from build123d import *

# Parameters (mm, degrees)
SKETCH1_R           = 38.1635
SKETCH1_R_2         = 13.716
BOSS_EXTRUDE3_DEPTH = 64.262
SKETCH3_R           = 38.1
SKETCH3_R_2         = 14.097
CUT_EXTRUDE1_DEPTH  = 62.23
FILLET1_R           = 2.54
SKETCH5_R           = 2.093695025
SKETCH5_R_2         = 2.032
SKETCH5_R_3         = 2.54
CUT_EXTRUDE2_DEPTH  = 2.54


with BuildPart() as part:
    # Sketch1 → Boss-Extrude3 (new body)
    with BuildSketch(Plane(origin=(0, 0, 0), x_dir=(1, 0, 0), z_dir=(0, 1, 0))):
        with Locations(Location((0, 0, 0), (0, 0, 270))):
            Circle(SKETCH1_R)
        with Locations(Location((0, 0, 0), (0, 0, 270))):
            Circle(SKETCH1_R_2, mode=Mode.SUBTRACT)
    extrude(amount=BOSS_EXTRUDE3_DEPTH)

    # Sketch3 → Cut-Extrude1 (cut)
    with BuildSketch(Plane(origin=(0, 0, 0), x_dir=(-1, 0, 0), z_dir=(0, -1, 0))):
        with Locations(Location((0, 0, 0), (0, 0, 90))):
            Circle(SKETCH3_R)
        with Locations(Location((0, 0, 0), (0, 0, 90))):
            Circle(SKETCH3_R_2, mode=Mode.SUBTRACT)
    extrude(amount=-CUT_EXTRUDE1_DEPTH, mode=Mode.SUBTRACT)

    # Fillet1
    fillet1_edges = [part.edges().sort_by_distance(p)[0] for p in [
        (0, 64.262, -38.1635),
        (0, 64.262, -13.716),
    ]]
    fillet(fillet1_edges, radius=FILLET1_R)

    # Sketch5 → Cut-Extrude2 (cut)
    with BuildSketch(Plane(origin=(0, 64.262, 0), x_dir=(1, 0, 0), z_dir=(0, 1, 0))):
        with Locations(Location((15.256423447, 20.307672038, 0), (0, 0, 270))):
            Circle(SKETCH5_R)
        with Locations(Location((-25.2151716, 3.058614257, 0), (0, 0, 270))):
            Circle(SKETCH5_R_2)
        with Locations(Location((9.958748153, -23.366286295, 0), (0, 0, 270))):
            Circle(SKETCH5_R_2)
        with Locations(Location((-9.958748153, 23.366286295, 0), (0, 0, 270))):
            Circle(SKETCH5_R_3)
    extrude(amount=-CUT_EXTRUDE2_DEPTH, mode=Mode.SUBTRACT)


solid = part.part
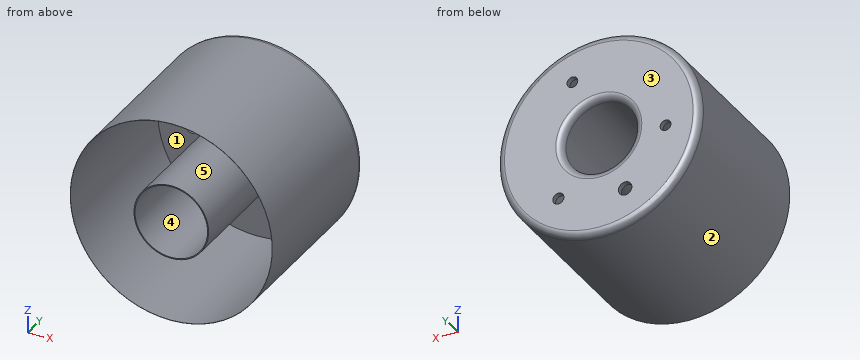
Check sheet for the modelled part. Datum: model origin and axes. Units: mm. Face numbers are marked on the shaded views. A direction names the side the tool comes from. Round coordinates to 2 decimals unless told otherwise and drop trailing zeros. Order: outer loops, then holes, each group sorted by start corner. A loop starts at its lowest first (then second) coordinate and runs counter-clockwise, first axis right, second up.
(1) Cross-section at B-B, the plane x = 0. Enter the section's corners in (y, z).
(2) Cross-section at A-A, the plane z = 0. Enter the section's corners in (x, y), and give its area (3 significant figures).
(3) Scan lines: probe 1 along Y at (x, z) = (26, 19); probe 2 along Z at (x, y) = (-35, 11). Record each from-to range of solid material in increasing order.
(4) Draft check along Z on the marked faces 1, 2 and 3. Enter one of: pulls with the +Z half, pulls with the -Z half, needs draft (parallel to the pull), parting line crosses it, or undercut.
(5) Go/stop test with flat-tipped pins: P1, Ø12, axis at x = -24.5, y = 34, coming from the -Z side; P2, Ø2, axis at x = 29.5, y = 6.5, coming from the -Z side; P3, Ø5, axis at x = -4, y = 45.5, coming from the +Z side. Record where each tip stops, or that it passes through.
(6) Cross-section at C-C, the plane y = 11.5. Enter the section's corners in (x, z).
(7) Access from +Z, -Z, +X, -X, +Y, -Y to the whole of each face (thin tool, end or side, straight path). Record for the marked faces 4 and 5.
Check sheet entries:
1. outline: (0, -38.16) - (61.72, -38.16) arc R2.54 ccw to (64.26, -35.62) - (64.26, -16.26) arc R2.54 ccw to (61.72, -13.72) - (0, -13.72) - (0, -14.1) - (62.23, -14.1) - (62.23, -38.1) - (0, -38.1) - close; (0, 13.72) - (61.72, 13.72) arc R2.54 ccw to (64.26, 16.26) - (64.26, 35.62) arc R2.54 ccw to (61.72, 38.16) - (0, 38.16) - (0, 38.1) - (62.23, 38.1) - (62.23, 14.1) - (0, 14.1) - close
2. outline: (-38.16, 0) - (-38.1, 0) - (-38.1, 62.23) - (-14.1, 62.23) - (-14.1, 0) - (-13.72, 0) - (-13.72, 61.72) arc R2.54 ccw to (-16.26, 64.26) - (-35.62, 64.26) arc R2.54 ccw to (-38.16, 61.72) - close; (13.72, 0) - (14.1, 0) - (14.1, 62.23) - (38.1, 62.23) - (38.1, 0) - (38.16, 0) - (38.16, 61.72) arc R2.54 ccw to (35.62, 64.26) - (16.26, 64.26) arc R2.54 ccw to (13.72, 61.72) - close
2. area: 149 mm2
3. probe 1: y = 62.23 to 64.26
3. probe 2: z = -15.21 to -15.05, 15.05 to 15.21
4. face 1: undercut
4. face 2: parting line crosses it
4. face 3: needs draft
5. P1: stops at z = -33.38
5. P2: stops at z = -25.38
5. P3: stops at z = 38.13
6. outline: circle Ø76.33 at (0, 0); circle Ø28.19 at (0, 0); hole circle Ø76.2 at (0, 0); hole circle Ø27.43 at (0, 0)
7. face 4: +Y, -Y
7. face 5: -Y
